The listing builds one solid part. Answer for the finished solid, in the listing's coordinates (mm). A direction names the side the tool comes from. Give positions to 0.01 mm unless a question says otherwise; leave off trailing zeros. Write each loop counter-clockwise with the first axis right and the second up, starting at its lowest first coordinate (ties: lowest second). Pieces come first, ordered by that corner, then holes.
```python
from build123d import *

# Parameters (mm, degrees)
PAD_DEPTH       = 120
FILLET_R        = 15
FILLET001_R     = 10
SKETCH001_R     = 20
PAD001_DEPTH    = 40
SKETCH002_R     = 10
POCKET_DEPTH    = 40
PAD002_DEPTH    = 8
SKETCH004_R     = 10
POCKET001_DEPTH = 8
PAD003_DEPTH    = 8
SKETCH006_R     = 10
POCKET002_DEPTH = 8
PAD004_DEPTH    = 8
SKETCH008_R     = 10
POCKET003_DEPTH = 8


with BuildPart() as part:
    # Sketch → Pad (new body)
    with BuildSketch(Plane.XY):
        Polygon((-39.5, 50), (-39.5, -40), (200.5, -40), (200.5, 30), (160.5, 30), (160.5, 0), (0.5, 0), (0.5, 50), align=None)
    extrude(amount=PAD_DEPTH)

    # Fillet
    fillet_edges = [part.edges().sort_by_distance(p)[0] for p in [
        (-39.5, 50, 60),
    ]]
    fillet(fillet_edges, radius=FILLET_R)

    # Fillet001
    fillet001_edges = [part.edges().sort_by_distance(p)[0] for p in [
        (180.5, 30, 120),
        (180.5, 30, 0),
    ]]
    fillet(fillet001_edges, radius=FILLET001_R)

    # Sketch001 (on Face2 of Fillet001) → Pad001 (join)
    with BuildSketch(Plane.YZ.offset(200.5)):
        with Locations((30, 60)):
            Circle(SKETCH001_R)
    extrude(amount=-PAD001_DEPTH)

    # Sketch002 (on Face12 of Pad001) → Pocket (cut)
    with BuildSketch(Plane.YZ.offset(200.5)):
        with Locations((30, 60)):
            Circle(SKETCH002_R)
    extrude(amount=-POCKET_DEPTH, mode=Mode.SUBTRACT)

    # Sketch003 (on Face4 of Pocket) → Pad002 (join)
    with BuildSketch(Plane.XZ.offset(40)):
        with BuildLine():
            Line((20.5, 140.000001), (20.5, 120))
            Line((20.5, 120), (-39.5, 120))
            Line((-39.5, 120), (-39.5, 140))
            ThreePointArc((20.5, 140.000001), (-9.5, 170), (-39.5, 140))
        make_face()
    extrude(amount=-PAD002_DEPTH)

    # Sketch004 (on Face16 of Pad002) → Pocket001 (cut)
    with BuildSketch(Plane.XZ.offset(40)):
        with Locations((-9.5, 140)):
            Circle(SKETCH004_R)
    extrude(amount=-POCKET001_DEPTH, mode=Mode.SUBTRACT)

    # Sketch005 (on Face4 of Pocket001) → Pad003 (join)
    with BuildSketch(Plane.XZ.offset(40)):
        with BuildLine():
            Line((200.5, 140), (200.5, 120))
            Line((200.5, 120), (140.5, 120))
            Line((140.5, 120), (140.5, 139.999999))
            ThreePointArc((200.5, 140), (170.5, 169.999999), (140.5, 139.999999))
        make_face()
    extrude(amount=-PAD003_DEPTH)

    # Sketch006 (on Face18 of Pad003) → Pocket002 (cut)
    with BuildSketch(Plane.XZ.offset(40)):
        with Locations((170.5, 139.999999)):
            Circle(SKETCH006_R)
    extrude(amount=-POCKET002_DEPTH, mode=Mode.SUBTRACT)

    # Sketch007 (on Face4 of Pocket002) → Pad004 (join)
    with BuildSketch(Plane.XZ.offset(40)):
        with BuildLine():
            Line((-39.5, 0), (20.5, 0))
            Line((20.5, 0), (20.5, -20))
            ThreePointArc((-39.5, -20), (-9.5, -50), (20.5, -20))
            Line((-39.5, -20), (-39.5, 0))
        make_face()
        with BuildLine():
            Line((140.5, 0), (200.5, 0))
            Line((200.5, 0), (200.5, -20))
            ThreePointArc((140.5, -20), (170.5, -49.99997), (200.5, -20))
            Line((140.5, -20), (140.5, 0))
        make_face()
    extrude(amount=-PAD004_DEPTH)

    # Sketch008 (on Face4 of Pad004) → Pocket003 (cut)
    with BuildSketch(Plane.XZ.offset(40)):
        with Locations((-9.5, -20)):
            Circle(SKETCH008_R)
        with Locations((170.5, -19.99997)):
            Circle(SKETCH008_R)
    extrude(amount=-POCKET003_DEPTH, mode=Mode.SUBTRACT)


solid = part.part
```
Item 1: A cutting plane is placed at D-D, the plane y = 26. Give the vertices of the cut face in (x, z), plus the area to 3 significant figures.
Conclusion:
outline: (-39.5, 0) - (0.5, 0) - (0.5, 120) - (-39.5, 120) - close; (160.5, 2) - (200.5, 2) - (200.5, 50.83) - (160.5, 50.83) - close; (160.5, 69.17) - (200.5, 69.17) - (200.5, 118) - (160.5, 118) - close
area: 8,710 mm2
Item 2: A cutting plane is placed at B-B, the plane x = 170.5. Give the vertices of the cut face in (y, z).
Conclusion:
outline: (-40, -50) - (-32, -50) - (-32, -30) - (-40, -30) - close; (-40, -10) - (-32, -10) - (-32, 0) - (20, 0) arc R10 ccw to (30, 10) - (30, 40) arc R20 ccw to (30, 80) - (30, 110) arc R10 ccw to (20, 120) - (-32, 120) - (-32, 130) - (-40, 130) - close; (-40, 150) - (-32, 150) - (-32, 170) - (-40, 170) - close; hole circle Ø20 at (30, 60)
Item 3: Consider probe 1 along Z at (x, y) = (170, -37); probe 2 along X at (y, z) = (5, 56); probe 3 along Y at (x, z) = (-28, 157). Determine where each line is inside the solid, lowest interval first.
Conclusion:
probe 1: z = -50 to -29.99, -10.01 to 130.01, 149.99 to 170
probe 2: x = -39.5 to 0.5, 160.5 to 200.5
probe 3: y = -40 to -32
Item 4: Which of the six approach directions +Z, -Z, +X, -X, +Y, -Y give full straight-line access (tool end or side, diameter ignored) to faces 1 (the face through (20.5, -36, 130)), 2 (the face through (160.5, 19, 61)), 3 (the face through (171, -32, 151))?
Conclusion:
face 1: +Z, +Y, -Y
face 2: +Z, -Z, +Y
face 3: +Z, +X, -X, +Y
Item 5: A cutting plane is placed at A-A, the plane z = 60. Give the vertices of the cut face in (x, y), plus the area to 3 significant figures.
Conclusion:
outline: (-39.5, -40) - (200.5, -40) - (200.5, 20) - (160.5, 20) - (160.5, 0) - (0.5, 0) - (0.5, 50) - (-24.5, 50) arc R15 ccw to (-39.5, 35) - close; (160.5, 40) - (200.5, 40) - (200.5, 50) - (160.5, 50) - close
area: 12,800 mm2
Item 6: Determine the mould class of faces 4 (the face through (-8.84, -36.056, 169.993)), 5 (the face through (175.114, -36.056, 131.128)), 6 (the face through (-11.67, -36.06, 130.24)), 7 (the face through (-9.1, -32, -30.2)) for opening direction Z: pulls with the +Z half, pulls with the -Z half, needs draft (parallel to the pull), parting line crosses it, or undercut.
Conclusion:
face 4: pulls with the +Z half
face 5: undercut
face 6: undercut
face 7: needs draft
Item 7: Each of these flat-tipped pins is pushed along its axis until it touches: P1, Ø24, axis at x = 186, z = 19.5, coming from the +Y side; P2, Ø2, axis at x = 30, z = 21.5, coming from the +Y side; P3, Ø4, axis at x = 148, y = -14, coming from the -Z side; P4, Ø18, axis at x = -9.5, z = 140, coming from the +Y side. Where does it stop, or does it pass through?
Conclusion:
P1: stops at y = 30
P2: stops at y = 0
P3: stops at z = 0
P4: passes through
Item 8: A cutting plane is placed at C-C, the plane y = 12. Give the vertices of the cut face in (x, z).
Conclusion:
outline: (-39.5, 0) - (0.5, 0) - (0.5, 120) - (-39.5, 120) - close; (160.5, 0) - (200.5, 0) - (200.5, 120) - (160.5, 120) - close
